from build123d import *

# Parameters (mm, degrees)
SKETCH2_OUTSIDE_W  = 28.352
SKETCH2_OUTSIDE_H  = 28.352
CUT_EXTRUDE1_DEPTH = 6


with BuildPart() as part:
    # Sketch1 → Revolve1 (revolve)
    with BuildSketch(Plane(origin=(0, 0, 0), x_dir=(0, 0, -1), z_dir=(1, 0, 0)), mode=Mode.PRIVATE) as revolve1_sk:
        Polygon((-8.1, 0), (-8.1, 9), (0, 9), (0, 4), (25, 4), (25, 0), align=None)
    revolve(revolve1_sk.sketch.rotate(Axis((0, 0, 5.584882278), (0, 0, -1)), 180), axis=Axis((0, 0, 5.584882278), (0, 0, -1)))

    # Sketch2 outside → Cut-Extrude1 (cut)
    with BuildSketch(Plane.XY.offset(8.1)):
        Rectangle(SKETCH2_OUTSIDE_W, SKETCH2_OUTSIDE_H)
        Polygon((3.75277675, -6.5), (7.505553499, 0), (3.75277675, 6.5), (-3.75277675, 6.5), (-7.505553499, 0), (-3.75277675, -6.5), align=None, mode=Mode.SUBTRACT)
    extrude(amount=-CUT_EXTRUDE1_DEPTH, mode=Mode.SUBTRACT)


solid = part.part
For this review, take the finished solid that the model builds, in its own axes (mm). A direction names the side the tool comes from. Coordinates: 2 decimals unless noted, no trailing zeros. Loops run counter-clockwise (first coordinate to the right, second up) from the corner with the lowest first, then second, coordinate; pieces in that order, holes last. Notation, with made-up numbers: (69.25, 81.5) - (107.25, 81.5) arc R18 ccw to (107.25, 112.5) - close; hole circle Ø1 at (25, 34). An arc over 180 degrees is marked (long way). Return JSON: item names as keys, results as strings.
Item 1: For faces 1 (the flat face through (-5.66, -3.2, 5.14)), 2 (the flat face through (0, 6.5, 5)), 3 (the flat face through (0, -7, 2.1)), 4 (the flat face through (5.6, -3.3, 5.1)), 5 (the flat face through (-5.6, 3.3, 5.1)), list the 3-axis set-ups (+Z, -Z, +X, -X, +Y, -Y) from which the entire face can be reached by the end or side of a thin tool; tool diameter is ignored.
Determined:
{"face 1": "+Z, -X, -Y", "face 2": "+Z, +X, -X, +Y", "face 3": "+Z", "face 4": "+Z, +X, -Y", "face 5": "+Z, -X, +Y"}
Item 2: Take a section at D-D (x = -6). Give the boundary of the cut face in (y, z).
Determined:
{"outline": "(-6.71, 0) - (6.71, 0) - (6.71, 2.1) - (2.61, 2.1) - (2.61, 8.1) - (-2.61, 8.1) - (-2.61, 2.1) - (-6.71, 2.1) - close"}
Item 3: Take a section at A-A (x = 0). Give the boundary of the cut face in (y, z), then the cut area to 3 significant figures.
Determined:
{"outline": "(-9, 0) - (-4, 0) - (-4, -25) - (4, -25) - (4, 0) - (9, 0) - (9, 2.1) - (6.5, 2.1) - (6.5, 8.1) - (-6.5, 8.1) - (-6.5, 2.1) - (-9, 2.1) - close", "area": "316 mm2"}
Item 4: Take a section at B-B (z = 2.5). Give the boundary of the cut face in (x, y).
Determined:
{"outline": "(-7.51, 0) - (-3.75, -6.5) - (3.75, -6.5) - (7.51, 0) - (3.75, 6.5) - (-3.75, 6.5) - close"}
Item 5: Take a section at C-C (y = -2). Give the boundary of the cut face in (x, z), then the cut area to 3 significant figures.
Determined:
{"outline": "(-8.77, 0) - (-3.46, 0) - (-3.46, -25) - (3.46, -25) - (3.46, 0) - (8.77, 0) - (8.77, 2.1) - (6.35, 2.1) - (6.35, 8.1) - (-6.35, 8.1) - (-6.35, 2.1) - (-8.77, 2.1) - close", "area": "286 mm2"}
Item 6: For line 1 (Z direction, x = 1.75, y = -7); line 2 (Z direction, x = 3.5, y = -2); line 3 (Y direction, x = 2.25, z = 3), list the stretches that pass through material, from the lowest coordinate up.
Determined:
{"line 1": "z = 0 to 2.1", "line 2": "z = 0 to 8.1", "line 3": "y = -6.5 to 6.5"}
Item 7: Insertion check: pin 1 (2 mm diameter, centred on x = -6, y = 3.5, fed in from -Z); pin 2 (4 mm diameter, centred on y = 1.5, z = -20.5, fed in from -X); pin 3 (8 mm diameter, centred on x = -5.5, z = -16, fed in from +Y); pin 4 (1 mm diameter, centred on y = -6, z = -4.5, fed in from -X). Each pin has a flat end and moves straight along its axis. Give the tip position at first contact, or say it passes through.
Determined:
{"pin 1": "stops at z = 0", "pin 2": "stops at x = -4", "pin 3": "stops at y = 3.71", "pin 4": "passes through"}
